```python
from build123d import *

# Parameters (mm, degrees)
BOSS_EXTRU_1_CORPS_DEPTH    = 310
CONG_1_R                    = 1.5
CONG_2_R                    = 0.4
CONG_4_R                    = 1
CONG_1_OF_SYM_TRIE_BRAS_R   = 1.5
CONG_2_OF_SYM_TRIE_BRAS_R   = 0.4
CONG_4_OF_SYM_TRIE_BRAS_R   = 1
SYM_TRIE_BRAS_DOUBLE_DEPTH  = 310
APR_S_TARODAGE_M6_R         = 3
ENL_V_MAT_FILETAGE_M6_DEPTH = 311.322412984


# Read off the part's stored shape, not the designer's step: Symétrie Bras double
with BuildPart() as part:
    # Esquisse4 → Boss.-Extru.1 Corps (new body)
    with BuildSketch(Plane(origin=(0, 0, 0), x_dir=(1, 0, 0), z_dir=(0, 1, 0))):
        Polygon((0, 0), (-4.5, 0), (-4.5, 3.625), (-6.875, 6), (-8.5, 6), (-8.5, 3), (-9.5, 3), (-9.5, 3.5), (-10, 3.5), (-10, 10), (-3.5, 10), (-3.5, 9.5), (-3, 9.5), (-3, 8.5), (-6, 8.5), (-6, 6.875), (-3.625, 4.5), (0, 4.5), align=None)
    boss_extru_1_corps = extrude(amount=BOSS_EXTRU_1_CORPS_DEPTH)

    # Congé1
    cong_1_edges = [part.edges().sort_by_distance(p)[0] for p in [
        (-10, 155, -10),
    ]]
    fillet(cong_1_edges, radius=CONG_1_R)

    # Congé2
    cong_2_edges = [part.edges().sort_by_distance(p)[0] for p in [
        (-8.5, 155, -6),
        (-6, 155, -8.5),
    ]]
    fillet(cong_2_edges, radius=CONG_2_R)

    # Congé4
    cong_4_edges = [part.edges().sort_by_distance(p)[0] for p in [
        (-4.5, 155, -3.625),
        (-6.875, 155, -6),
        (-6, 155, -6.875),
        (-3.625, 155, -4.5),
    ]]
    fillet(cong_4_edges, radius=CONG_4_R)

    # Symétrie Bras: Boss.-Extru.1 Corps across plane
    add(boss_extru_1_corps.mirror(Plane(origin=(0, 310, -4.5), x_dir=(0, 0, 1), z_dir=(-1, 0, 0))))

    # Congé1 of Symétrie Bras
    cong_1_of_sym_trie_bras_edges = [part.edges().sort_by_distance(p)[0] for p in [
        (10, 155, -10),
    ]]
    fillet(cong_1_of_sym_trie_bras_edges, radius=CONG_1_OF_SYM_TRIE_BRAS_R)

    # Congé2 of Symétrie Bras
    cong_2_of_sym_trie_bras_edges = [part.edges().sort_by_distance(p)[0] for p in [
        (8.5, 155, -6),
        (6, 155, -8.5),
    ]]
    fillet(cong_2_of_sym_trie_bras_edges, radius=CONG_2_OF_SYM_TRIE_BRAS_R)

    # Congé4 of Symétrie Bras
    cong_4_of_sym_trie_bras_edges = [part.edges().sort_by_distance(p)[0] for p in [
        (4.5, 155, -3.625),
        (6.875, 155, -6),
        (6, 155, -6.875),
        (3.625, 155, -4.5),
    ]]
    fillet(cong_4_of_sym_trie_bras_edges, radius=CONG_4_OF_SYM_TRIE_BRAS_R)

    # Symétrie Bras double outline → Symétrie Bras double (add)
    with BuildSketch(Plane(origin=(0, 0, 0), x_dir=(1, 0, 0), z_dir=(0, 1, 0))):
        with BuildLine():
            ThreePointArc((7.289213562, -6), (6.90653013, -5.923879533), (6.582106781, -5.707106781))
            Line((6.582106781, -5.707106781), (4.792893219, -3.917893219))
            ThreePointArc((4.792893219, -3.917893219), (4.576120467, -3.59346987), (4.5, -3.210786438))
            Line((4.5, -3.210786438), (4.5, 0))
            Line((4.5, 0), (-4.5, 0))
            Line((-4.5, 0), (-4.5, -3.210786438))
            ThreePointArc((-4.5, -3.210786438), (-4.576120467, -3.59346987), (-4.792893219, -3.917893219))
            Line((-4.792893219, -3.917893219), (-6.582106781, -5.707106781))
            ThreePointArc((-6.582106781, -5.707106781), (-6.90653013, -5.923879533), (-7.289213562, -6))
            Line((-7.289213562, -6), (-8.1, -6))
            ThreePointArc((-8.1, -6), (-8.382842712, -5.882842712), (-8.5, -5.6))
            Line((-8.5, -5.6), (-8.5, -3))
            Line((-8.5, -3), (-9.5, -3))
            Line((-9.5, -3), (-9.5, -3.5))
            Line((-9.5, -3.5), (-10, -3.5))
            Line((-10, -3.5), (-10, -8.5))
            ThreePointArc((-10, -8.5), (-9.560660172, -9.560660172), (-8.5, -10))
            Line((-8.5, -10), (-3.5, -10))
            Line((-3.5, -10), (-3.5, -9.5))
            Line((-3.5, -9.5), (-3, -9.5))
            Line((-3, -9.5), (-3, -8.5))
            Line((-3, -8.5), (-5.6, -8.5))
            ThreePointArc((-5.6, -8.5), (-5.882842712, -8.382842712), (-6, -8.1))
            Line((-6, -8.1), (-6, -7.289213562))
            ThreePointArc((-6, -7.289213562), (-5.923879533, -6.90653013), (-5.707106781, -6.582106781))
            Line((-5.707106781, -6.582106781), (-3.917893219, -4.792893219))
            ThreePointArc((-3.917893219, -4.792893219), (-3.59346987, -4.576120467), (-3.210786438, -4.5))
            Line((-3.210786438, -4.5), (3.210786438, -4.5))
            ThreePointArc((3.210786438, -4.5), (3.59346987, -4.576120467), (3.917893219, -4.792893219))
            Line((3.917893219, -4.792893219), (5.707106781, -6.582106781))
            ThreePointArc((5.707106781, -6.582106781), (5.923879533, -6.90653013), (6, -7.289213562))
            Line((6, -7.289213562), (6, -8.1))
            ThreePointArc((6, -8.1), (5.882842712, -8.382842712), (5.6, -8.5))
            Line((5.6, -8.5), (3, -8.5))
            Line((3, -8.5), (3, -9.5))
            Line((3, -9.5), (3.5, -9.5))
            Line((3.5, -9.5), (3.5, -10))
            Line((3.5, -10), (8.5, -10))
            ThreePointArc((8.5, -10), (9.560660172, -9.560660172), (10, -8.5))
            Line((10, -8.5), (10, -3.5))
            Line((10, -3.5), (9.5, -3.5))
            Line((9.5, -3.5), (9.5, -3))
            Line((9.5, -3), (8.5, -3))
            Line((8.5, -3), (8.5, -5.6))
            ThreePointArc((8.5, -5.6), (8.382842712, -5.882842712), (8.1, -6))
            Line((8.1, -6), (7.289213562, -6))
        make_face()
    extrude(amount=SYM_TRIE_BRAS_DOUBLE_DEPTH)

    # Après tarodage M6 → Enlèv. mat.-Filetage M6 (cut, through all)
    with BuildSketch(Plane.XZ):
        with Locations(Location((0, 0, 0), (0, 0, 270))):
            Circle(APR_S_TARODAGE_M6_R)
    extrude(amount=-ENL_V_MAT_FILETAGE_M6_DEPTH, mode=Mode.SUBTRACT)


solid = part.part
```
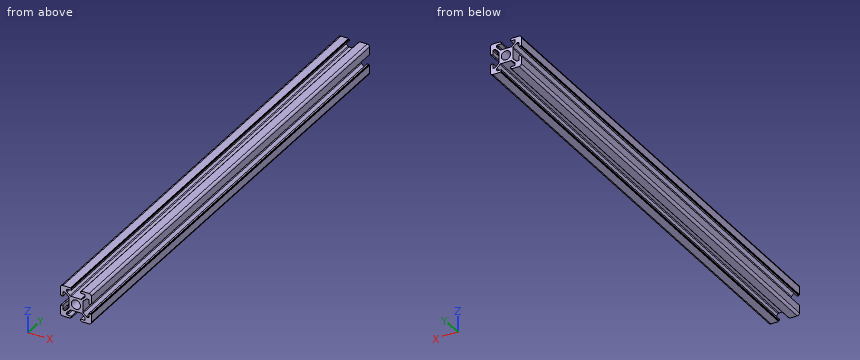
Verification items for the finished model (mm, model axes). Coordinates: 2 decimals unless noted, no trailing zeros. Write each loop counter-clockwise with the first axis right and the second up, starting at its lowest first coordinate (ties: lowest second). Pieces come first, ordered by that corner, then holes. Notation, with made-up numbers: M -39,22 L 8,22 A9 ccw 8,29 Z; hole C 36.25,89 d7. An arc over 180 degrees is marked long. One line per item, written item: value.
Item 1: Section check B-B, the plane x = 0. Record the boundary of the cut face in (y, z).
Check sheet entries:
outline: M 0,-4.5 L 310,-4.5 L 310,-3 L 0,-3 Z; M 0,3 L 310,3 L 310,4.5 L 0,4.5 Z
Item 2: Gauge pin test, flat ends, axial feed: pin 1 Ø3 at (x, z) = (0.5, -7.5) entering from +Y; pin 2 Ø3 at (x, y) = (0, 158.5) entering from +Z; pin 3 Ø0.5 at (y, z) = (107.5, -9) entering from +X; pin 4 Ø0.6 at (y, z) = (101.5, -9.5) entering from +X. Record the tip position at first contact, or that the pin passes through.
Check sheet entries:
pin 1: passes through
pin 2: stops at z = 4.5
pin 3: stops at x = 9.98
pin 4: stops at x = 9.83
Item 3: Scan lines: line 1 along X through (y, z) = (226, -7.25); line 2 along X through (y, z) = (96.5, 0); line 3 along X through (y, z) = (187.5, -5) (3 decimals). Record each from-to range of solid material in increasing order.
Check sheet entries:
line 1: x = -10 to -6, 6 to 10
line 2: x = -4.5 to -3, 3 to 4.5
line 3: x = -10 to -8.5, -5.875 to -4.125, 4.125 to 5.875, 8.5 to 10
Item 4: Section check A-A, the plane z = 0. Record the boundary of the cut face in (x, y), plus the area to 3 significant figures.
Check sheet entries:
outline: M -4.5,0 L -3,0 L -3,310 L -4.5,310 Z; M 3,0 L 4.5,0 L 4.5,310 L 3,310 Z
area: 930 mm^2
